Read the model definition and answer for the solid it produces. Units are mm, in the model's axes. A direction names the side the tool comes from. Coordinates: 2 decimals unless noted, no trailing zeros. Order: outer loops, then holes, each group sorted by start corner. A loop starts at its lowest first (then second) coordinate and runs counter-clockwise, first axis right, second up. Notation, with made-up numbers: (-39, 59.5) - (4, 59.5) arc R12 cw to (4, 80.5) - close; hole circle Ø5 at (76, 33). An arc over 180 degrees is marked (long way). Use one line per item in the form item = value.
```python
from build123d import *

# Parameters (mm, degrees)
F0_W        = 30.5091738701
F0_H        = 52.441470325
F1_DEPTH    = 10.5918
F3_DEPTH    = 1.778
F5_DEPTH    = 1.778
F6_T1_DEPTH = 30.5091738701
F6_T6_DEPTH = 49.8209621392
F7_R        = 2.54


# Not quite as in the source:
# - a fillet or chamfer that OpenCascade refuses, or shapes differently, is made with other operations: its cross-section is extruded or revolved along the edge and cut away or added


with BuildPart() as f1:
    # F0 (on Top) → F1 (new body)
    with BuildSketch(Plane.XY):
        with Locations((15.254586935, 26.2207351625)):
            Rectangle(F0_W, F0_H)
    extrude(amount=F1_DEPTH)

    # F2 (on face) → F3 (cut)
    with BuildSketch(Plane.XY.offset(10.5918)):
        Polygon((27.9714719847, 52.441470325), (0, 52.441470325), (0, 27.7975574136), (0, 26.2207351625), (30.5091738701, 26.2207351625), (30.5091738701, 52.4368782499), align=None)
    extrude(amount=-F3_DEPTH, mode=Mode.SUBTRACT)

    # F4 (on face) → F5 (cut)
    with BuildSketch(Plane(origin=(0, 0, 0), x_dir=(1, 0, 0), z_dir=(0, 0, -1))):
        Polygon((30.5091738701, -26.980528608), (0, -26.2207351625), (0, -52.441470325), (30.5091738701, -52.441470325), align=None)
    extrude(amount=-F5_DEPTH, mode=Mode.SUBTRACT)

    # F6: fillet of radius 5.08 on 2 edges, made by hand

    # F6_s2 → F6_t1 (join)
    with BuildSketch(Plane.YZ):
        with BuildLine():
            ThreePointArc((26.2207351625, 10.5918), (27.9560844701, 9.2796608604), (30.0812009375, 8.8138))
            Line((30.0812009375, 8.8138), (26.2207351625, 8.8138))
            Line((26.2207351625, 8.8138), (26.2207351625, 10.5918))
        make_face()
    extrude(amount=F6_T1_DEPTH)


with BuildPart() as f6_tool4:
    # F6_s5 → F6_t6 (new body)
    with BuildSketch(Plane(origin=(40.8099373033, 1.0163212877, 0), x_dir=(0, 0, 1), z_dir=(-0.9996900453, -0.0248960508, 0))):
        with BuildLine():
            ThreePointArc((1.778, 30.0730736971), (1.3121391396, 27.9479572297), (0, 26.2126079221))
            Line((0, 26.2126079221), (1.778, 26.2126079221))
            Line((1.778, 26.2126079221), (1.778, 30.0730736971))
        make_face()
    extrude(amount=F6_T6_DEPTH)

    split(bisect_by=Plane.YZ, keep=Keep.TOP)

    split(bisect_by=Plane.YZ.offset(30.5091738701), keep=Keep.BOTTOM)


with BuildPart() as f1_1:
    add(f1.part)

    # F6_t3: union F6_tool4
    add(f6_tool4.part)

    # F7
    f7_edges = [f1_1.edges().sort_by_distance(p)[0] for p in [
        (15.254587, 52.44147, 1.778),
        (15.254587, 0, 0),
        (15.254587, 0, 10.5918),
        (13.985736, 52.44147, 8.8138),
    ]]
    fillet(f7_edges, radius=F7_R)


solid = f1_1.part
```
(1) The mould has two halves that part along Y. Classify faces 4 (the flat face through (15, 52.441, 5)), 5 (the flat face through (15, 0, 5)), 6 (the flat face through (0, 26, 5)): +Y half, -Y half, draft (parallel to the pull), parting line (faces both ways), or undercut.
Answer list:
face_4 = +Y half
face_5 = -Y half
face_6 = draft
(2) Straight lines are drawn through the part: L1, parallel to Z at x = 17.5, y = 32; L2, parallel to Y at x = 15, z = 7.25; L3, parallel to Y at x = 7.5, z = 4.25. For each, find the intervals that lie inside material, in ascending order.
Answer list:
L1 = 1.78 to 8.81
L2 = 0 to 52.25
L3 = 0 to 52.44
(3) Section A-A, the plane y = 47.5 is taken. Write down the section's boundary in (x, z).
Answer list:
outline = (0, 1.78) - (30.51, 1.78) - (30.51, 8.81) - (0, 8.81) - close
(4) Which of the six approach directions +Z, -Z, +X, -X, +Y, -Y give full straight-line access (tool end or side, diameter ignored) to faces 1 (the flat face through (15, 40, 1.778)), 2 (the flat face through (15, 40, 8.814)), 3 (the cylindrical face through (15.473, 28.37, 1.325))?
Answer list:
face_1 = -Z, +X, -X, +Y
face_2 = +Z, +X, -X, +Y
face_3 = -Z, -X, +Y
(5) Given pin 1 Ø16 at (x, y) = (9.5, 38) entering from +Z; pin 2 Ø12 at (x, y) = (17, 41) entering from -Z; pin 3 Ø12 at (x, y) = (11, 33) entering from -Z, each flat-ended and moving along its own axis, determine where each tip first touches the part or whether it passes through.
Answer list:
pin_1 = 8.81
pin_2 = 1.78
pin_3 = 0.51
